Geometry check sheet. Reference: the model listing, model coordinates, mm. Face numbers are marked on the shaded views. Round coordinates to 2 decimals unless told otherwise and drop trailing zeros. Order: outer loops, then holes, each group sorted by start corner. A loop starts at its lowest first (then second) coordinate and runs counter-clockwise, first axis right, second up. Notation, with made-up numbers: (31.25, -39) - (61.25, -39) arc R9 cw to (61.25, -35) - close; hole circle Ø6 at (26.25, -29). An arc over 180 degrees is marked (long way). Use a Markdown table: item, result. Add a question column.
(1) Thickness scan on line 1 along Y through (x, z) = (-622.5, 425); line 2 along X through (y, z) = (-9, 822); line 3 along X through (y, z) = (54, 1098). Record the ranges inside material, lowest first. Write a range as [from, to].
(2) Gauge pin test, flat ends, axial feed: P1, Ø10, axis at y = 46.5, z = 238, coming from the +X side; P2, Ø1.5, axis at x = 699, z = 317.5, coming from the +Y side; P3, Ø10, axis at y = -102.5, z = 829, coming from the +X side. Record the tip position at first contact, or that the pin passes through.
(3) Section check C-C on x = -255. Record the boundary of the cut face in (y, z), then the cut area to 3 significant figures.
(4) Section check B-B on z = 182. Record the boundary of the cut face in (x, y).
(5) Section check A-A on y = 0. Record the boundary of the cut face in (x, z).
(6) Mould release check, pull along X, two halves, no side actions. Record for the marked faces 1 and 2: released by +X, released by -X, zero draft, split by the parting line, or undercut.
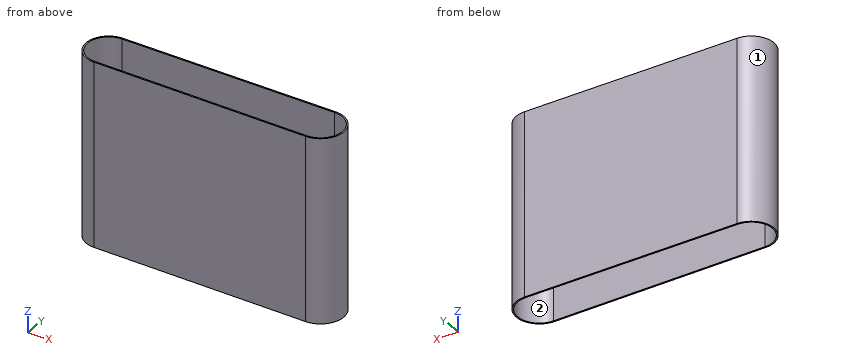
Autodesk Inventor part; units mm, degrees
ref_plane "YZ Plane" through (0, 0, 0) normal (1, 0, 0) x (0, 1, 0)
ref_plane "XZ Plane" through (0, 0, 0) normal (0, 1, 0) x (-1, 0, 0)
ref_plane "XY Plane" through (0, 0, 0) normal (0, 0, 1) x (1, 0, 0)
sketch "Boceto1" plane through (0, 0, 0) normal (0, 0, 1) x (1, 0, 0)
  arc A0 (-750.5267, 157.9991) -> (-750.5267, -157.9991) centre (-750, 0) ccw
  arc A1 (749.4567, -162.9991) -> (749.4567, 162.9991) centre (750, 0) ccw
  line L0 (-750.5267, 157.9991) -> (749.4567, 162.9991)
  line L1 (749.4567, -162.9991) -> (-750.5267, -157.9991)
  line L2 (749.49, 152.9991) -> (-750.4933, 147.9992)
  arc A2 (-750.4933, 147.9992) -> (-750.4933, -147.9992) centre (-750, 0) ccw
  line L3 (-750.4933, -147.9992) -> (749.49, -152.9991)
  arc A3 (749.49, -152.9991) -> (749.49, 152.9991) centre (750, 0) ccw
  point P0 (0, 0)
  dimension "d0" = 1500
  dimension "d1" = 326
  dimension "d2" = 316
  dimension "d3" = 750
  dimension "d4" = 10
extrude "Extrusión1" add sketch "Boceto1" along normal blind 1300
properties part number "faja"
Check sheet entries:
| question | item | result |
|---|---|---|
| 1 | line 1 | y = [-158.43, -148.43], [148.43, 158.43] |
| 1 | line 2 | x = [-907.74, -897.73], [902.74, 912.75] |
| 1 | line 3 | x = [-898.49, -887.8], [893.15, 903.8] |
| 2 | P1 | stops at x = 907.63 |
| 2 | P2 | stops at y = 162.83 |
| 2 | P3 | stops at x = 880.62 |
| 3 | outline | (-159.65, 0) - (-149.65, 0) - (-149.65, 1300) - (-159.65, 1300) - close; (149.65, 0) - (159.65, 0) - (159.65, 1300) - (149.65, 1300) - close |
| 3 | area | 26,000 mm2 |
| 4 | outline | (-750.53, -158) - (749.46, -163) arc R163 ccw (long way) to (749.46, 163) - (-750.53, 158) arc R158 ccw to start; hole (-750.49, -148) - (749.49, -153) arc R153 ccw (long way) to (749.49, 153) - (-750.49, 148) arc R148 ccw to start |
| 5 | outline | (-908, 0) - (-898, 0) - (-898, 1300) - (-908, 1300) - close; (903, 0) - (913, 0) - (913, 1300) - (903, 1300) - close |
| 6 | face 1 | released by -X |
| 6 | face 2 | undercut |
